Here's how the part is built. I have some questions about the finished solid (model axes, mm). A direction names the side the tool comes from. Round coordinates to 2 decimals unless told otherwise and drop trailing zeros. Write each loop counter-clockwise with the first axis right and the second up, starting at its lowest first coordinate (ties: lowest second). Pieces come first, ordered by that corner, then holes. Notation, with made-up numbers: (83.5, -36.75) - (113.5, -36.75) arc R19 ccw to (113.5, -16.75) - close; hole circle Ø10 at (24, 17). An arc over 180 degrees is marked (long way). Write item = value, one per line. Start each with the question number.
Item 1: If we section it at D-D (x = 13): Please give me the cut outline in (y, z).
Item 2: Thinking about a two-plate mould opening in Y: for faces 1 (the face through (31.91, 23.92, 74.26)), 2 (the face through (94.557, 58.492, 74.26)), 3 (the face through (60.39, 46.413, 74.24)), 4 (the face through (63, 36, 0)), which applies, pulls with the +Y half, pulls with the -Y half, needs draft (parallel to the pull), parting line crosses it, or undercut?
Item 3: If we section it at C-C (y = 20.5): Please give me the cut outline in (x, z).
Item 4: If I drill on line 1 along Z through (x, y) = (47, 28); line 2 along Y through (x, z) = (36.5, 42); line 3 along X through (y, z) = (32.5, 63.5), over which ranges is the centre line in solid material (lowest first)? Write a range as [from, to].
Item 5: For P1, Ø1.5, axis at y = 12.5, z = 33, coming from the +X side; P2, Ø5, axis at y = 34, z = 66, coming from the +X side; P3, Ø3.5, axis at x = 93.81, y = 59.93, coming from the -Z side, each with a flat end and sliding along its axis, tell me the tip position at first contact or that it passes through.
Item 6: If we section it at A-A (z = 42): Please give me the cut outline in (x, y) (3 decimals).
Item 7: Which directions (+Z, -Z, +X, -X, +Y, -Y) give clear straight access to the entire face, cutting with the end or side of a thin tool? Please do faces 5 (the face through (57.67, 29.83, 36.98)), 6 (the face through (63, 42, 73.5)), 7 (the face through (20.23, 17.37, 74.26)).
Item 8: If we section it at B-B (x = 101): Please give me the cut outline in (y, z).
```python
from build123d import *

# Parameters (mm, degrees)
BOSS_EXTRUDE1_DEPTH = 75
SKETCH2_W           = 100
SKETCH2_H           = 1.5
BOSS_EXTRUDE2_DEPTH = 10
SKETCH3_R           = 1.625
CUT_EXTRUDE1_DEPTH  = 152.825931424


with BuildPart() as part:
    # Sketch1 → Boss-Extrude1 (new body)
    with BuildSketch(Plane.XY):
        Polygon((0, 0), (6, 0), (110.797734112, 60.505), (109.297734112, 63.103076211), align=None)
    extrude(amount=BOSS_EXTRUDE1_DEPTH)

    # Sketch2 → Boss-Extrude2 (add)
    with BuildSketch(Plane(origin=(0, 0, 0), x_dir=(0.866025403784438, 0.5000000000000012, 0), z_dir=(-0.5000000000000011, 0.8660254037844379, 0))):
        with Locations((76.206152423, -74.25)):
            Rectangle(SKETCH2_W, SKETCH2_H)
    extrude(amount=BOSS_EXTRUDE2_DEPTH)

    # Sketch3 → Cut-Extrude1 (cut, through all)
    with BuildSketch(Plane.XY.offset(75)):
        with Locations((33.198138972, 24.911441429)):
            Circle(SKETCH3_R)
        with Locations((93.807353055, 59.93320323)):
            Circle(SKETCH3_R)
    extrude(amount=-CUT_EXTRUDE1_DEPTH, mode=Mode.SUBTRACT)


solid = part.part
```
Reply:
q1.outline = (4.04, 0) - (7.51, 0) - (7.51, 75) - (4.04, 75) - close
q2.face_1 = undercut
q2.face_2 = undercut
q2.face_3 = pulls with the +Y half
q2.face_4 = needs draft
q3.outline = (18.42, 73.5) - (35.51, 73.5) - (35.51, 0) - (41.51, 0) - (41.51, 75) - (18.42, 75) - close
q4.line_1 = [73.5, 75]
q4.line_2 = [17.61, 21.07]
q4.line_3 = [56.29, 62.29]
q5.P1 = 28.95
q5.P2 = 69.22
q5.P3 = 73.5
q6.outline = (0, 0) - (6, 0) - (110.798, 60.505) - (109.298, 63.103) - close
q7.face_5 = +Z, -Z, +X, -Y
q7.face_6 = -Z, -X, +Y
q7.face_7 = +Z, -Z, -X
q8.outline = (54.85, 0) - (58.31, 0) - (58.31, 73.5) - (69.86, 73.5) - (69.86, 75) - (54.85, 75) - close
